Verification items for the finished model (mm, model axes). Face numbers are marked on the shaded views. A direction names the side the tool comes from. Coordinates: 2 decimals unless noted, no trailing zeros. Write each loop counter-clockwise with the first axis right and the second up, starting at its lowest first coordinate (ties: lowest second). Pieces come first, ordered by that corner, then holes.
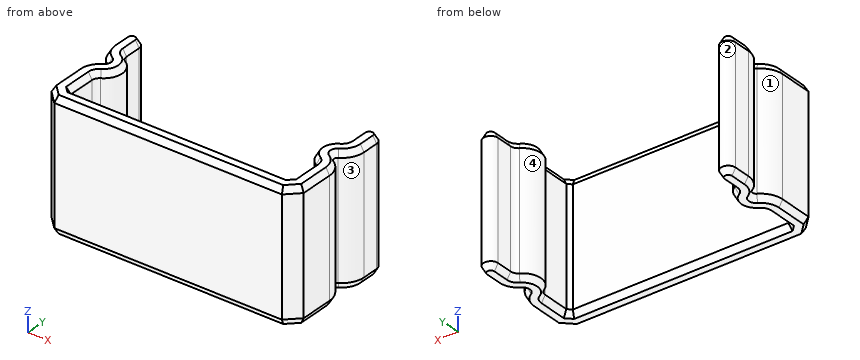
```python
from build123d import *

# Parameters (mm, degrees)
BOSS_EXTRUDE1_DEPTH   = 7
CHAMFER1_SIZE         = 0.2
CHAMFER1_SIZE2        = 0.346410162
CHAMFER1_PART_2_SIZE  = 0.2
CHAMFER1_PART_2_SIZE2 = 0.346410162


with BuildPart() as part:
    # Sketch1 → Boss-Extrude1 (new body)
    with BuildSketch(Plane.XY):
        with BuildLine():
            Line((5.85, 0), (-5.85, 0))
            Line((-5.85, 0), (-6.05, 0.2))
            Line((-6.05, 0.2), (-6.05, 1.687564435))
            ThreePointArc((-6.05, 1.687564435), (-5.996410162, 1.887564435), (-5.85, 2.033974596))
            ThreePointArc((-5.85, 2.033974596), (-5.35, 2.9), (-5.85, 3.766025404))
            ThreePointArc((-5.85, 3.766025404), (-5.996410162, 3.912435565), (-6.05, 4.112435565))
            Line((-6.05, 4.112435565), (-6.05, 5))
            ThreePointArc((-6.05, 5), (-6.45, 5.4), (-6.85, 5))
            Line((-6.85, 5), (-6.85, 4.112435565))
            ThreePointArc((-6.85, 4.112435565), (-6.689230485, 3.512435565), (-6.25, 3.073205081))
            ThreePointArc((-6.25, 3.073205081), (-6.15, 2.9), (-6.25, 2.726794919))
            ThreePointArc((-6.25, 2.726794919), (-6.689230485, 2.287564435), (-6.85, 1.687564435))
            Line((-6.85, 1.687564435), (-6.85, -0.13137085))
            Line((-6.85, -0.13137085), (-6.18137085, -0.8))
            Line((-6.18137085, -0.8), (6.18137085, -0.8))
            Line((6.18137085, -0.8), (6.85, -0.13137085))
            Line((6.85, -0.13137085), (6.85, 1.687564435))
            ThreePointArc((6.85, 1.687564435), (6.689230485, 2.287564435), (6.25, 2.726794919))
            ThreePointArc((6.25, 2.726794919), (6.15, 2.9), (6.25, 3.073205081))
            ThreePointArc((6.25, 3.073205081), (6.689230485, 3.512435565), (6.85, 4.112435565))
            Line((6.85, 4.112435565), (6.85, 5))
            ThreePointArc((6.85, 5), (6.45, 5.4), (6.05, 5))
            Line((6.05, 5), (6.05, 4.112435565))
            ThreePointArc((6.05, 4.112435565), (5.996410162, 3.912435565), (5.85, 3.766025404))
            ThreePointArc((5.85, 3.766025404), (5.35, 2.9), (5.85, 2.033974596))
            ThreePointArc((5.85, 2.033974596), (5.996410162, 1.887564435), (6.05, 1.687564435))
            Line((6.05, 1.687564435), (6.05, 0.2))
            Line((6.05, 0.2), (5.85, 0))
        make_face()
    extrude(amount=BOSS_EXTRUDE1_DEPTH)

    # Chamfer1
    chamfer1_edges = [part.edges().sort_by_distance(p)[0] for p in [
        (5.95, 0.1, 7),
        (0, 0, 7),
        (-5.95, 0.1, 7),
        (-6.05, 0.943782217, 7),
        (-5.996410162, 3.912435565, 7),
        (-6.05, 4.556217783, 7),
        (-6.45, 5.4, 7),
        (-6.85, 4.556217783, 7),
        (-6.689230485, 3.512435565, 7),
        (-6.15, 2.9, 7),
        (-6.689230485, 2.287564435, 7),
        (-6.85, 0.778096792, 7),
        (-6.515685425, -0.465685425, 7),
        (0, -0.8, 7),
        (-5.996410162, 1.887564435, 7),
        (6.515685425, -0.465685425, 7),
        (6.85, 0.778096792, 7),
        (6.689230485, 2.287564435, 7),
        (6.15, 2.9, 7),
        (6.689230485, 3.512435565, 7),
        (6.85, 4.556217783, 7),
        (6.45, 5.4, 7),
        (6.05, 4.556217783, 7),
        (5.996410162, 3.912435565, 7),
        (5.35, 2.9, 7),
        (-5.35, 2.9, 7),
        (5.996410162, 1.887564435, 7),
        (6.05, 0.943782217, 7),
    ]]
    chamfer1_side = [part.faces().sort_by_distance(p)[0] for p in [
        (6.126639766, 1.962752532, 7),
    ]]
    chamfer(chamfer1_edges, length=CHAMFER1_SIZE, length2=CHAMFER1_SIZE2, reference=chamfer1_side[0])

    # Chamfer1 part 2
    chamfer1_part_2_edges = [part.edges().sort_by_distance(p)[0] for p in [
        (-6.05, 0.943782217, 0),
        (-5.95, 0.1, 0),
        (0, 0, 0),
        (5.95, 0.1, 0),
        (6.05, 0.943782217, 0),
        (5.996410162, 1.887564435, 0),
        (5.35, 2.9, 0),
        (5.996410162, 3.912435565, 0),
        (6.05, 4.556217783, 0),
        (6.45, 5.4, 0),
        (6.85, 4.556217783, 0),
        (6.689230485, 3.512435565, 0),
        (6.15, 2.9, 0),
        (6.689230485, 2.287564435, 0),
        (6.85, 0.778096792, 0),
        (6.515685425, -0.465685425, 0),
        (0, -0.8, 0),
        (-6.515685425, -0.465685425, 0),
        (-6.85, 0.778096792, 0),
        (-6.689230485, 2.287564435, 0),
        (-6.15, 2.9, 0),
        (-6.689230485, 3.512435565, 0),
        (-6.85, 4.556217783, 0),
        (-6.45, 5.4, 0),
        (-6.05, 4.556217783, 0),
        (-5.996410162, 3.912435565, 0),
        (-5.35, 2.9, 0),
        (-5.996410162, 1.887564435, 0),
    ]]
    chamfer1_part_2_side = [part.faces().sort_by_distance(p)[0] for p in [
        (6.126639766, 1.962752532, 0),
    ]]
    chamfer(chamfer1_part_2_edges, length=CHAMFER1_PART_2_SIZE, length2=CHAMFER1_PART_2_SIZE2, reference=chamfer1_part_2_side[0])


solid = part.part
```
1. Sectioned sample at B-B, the plane y = 4.75. Record the boundary of the cut face in (x, z), and give its area (3 significant figures).
2. Tool access check on the marked faces 1, 2, 3 and 4. Record the directions out of +Z, -Z, +X, -X, +Y, -Y that give a thin tool (end or side, any length) a straight path to the whole face; none if there is none.
3. Sectioned sample at C-C, the plane x = 3.5. Record the boundary of the cut face in (y, z).
4. Gauge pin test, flat ends, axial feed: P1, Ø2, axis at x = 1.5, y = 2, coming from the +Z side; P2, Ø3, axis at y = 3, z = 4, coming from the +X side; P3, Ø3, axis at x = 2, z = 4, coming from the +Y side. Record the tip position at first contact, or that the pin passes through.
5. Material ranges on L1, parallel to X at y = 1.25, z = 5.75; L2, parallel to Y at x = 3.5, z = 5; L3, parallel to X at y = 2.25, z = 2.5, recorded low to high.
6. Sectioned sample at A-A, the plane z = 1.5. Record the boundary of the cut face in (x, y).
Outcome:
1. outline: (-6.85, 0.35) - (-6.65, 0) - (-6.25, 0) - (-6.05, 0.35) - (-6.05, 6.65) - (-6.25, 7) - (-6.65, 7) - (-6.85, 6.65) - close; (6.05, 0.35) - (6.25, 0) - (6.65, 0) - (6.85, 0.35) - (6.85, 6.65) - (6.65, 7) - (6.25, 7) - (6.05, 6.65) - close
1. area: 10.9 mm2
2. face 1: +Z, -Z, -X
2. face 2: +Z, -Z, +Y
2. face 3: +Z, -Z, +X
2. face 4: +Z, -Z
3. outline: (-0.8, 0.35) - (-0.6, 0) - (-0.2, 0) - (0, 0.35) - (0, 6.65) - (-0.2, 7) - (-0.6, 7) - (-0.8, 6.65) - close
4. P1: passes through
4. P2: stops at x = 6.85
4. P3: stops at y = 0
5. L1: x = -6.85 to -6.05, 6.05 to 6.85
5. L2: y = -0.8 to 0
5. L3: x = -6.71 to -5.59, 5.59 to 6.71
6. outline: (-6.85, -0.13) - (-6.18, -0.8) - (6.18, -0.8) - (6.85, -0.13) - (6.85, 1.69) arc R1.2 ccw to (6.25, 2.73) arc R0.2 cw to (6.25, 3.07) arc R1.2 ccw to (6.85, 4.11) - (6.85, 5) arc R0.4 ccw to (6.05, 5) - (6.05, 4.11) arc R0.4 cw to (5.85, 3.77) arc R1 ccw to (5.85, 2.03) arc R0.4 cw to (6.05, 1.69) - (6.05, 0.2) - (5.85, 0) - (-5.85, 0) - (-6.05, 0.2) - (-6.05, 1.69) arc R0.4 cw to (-5.85, 2.03) arc R1 ccw to (-5.85, 3.77) arc R0.4 cw to (-6.05, 4.11) - (-6.05, 5) arc R0.4 ccw to (-6.85, 5) - (-6.85, 4.11) arc R1.2 ccw to (-6.25, 3.07) arc R0.2 cw to (-6.25, 2.73) arc R1.2 ccw to (-6.85, 1.69) - close
